Here's how the part is built. I have some questions about the finished solid (model axes, mm). Round coordinates to 2 decimals unless told otherwise and drop trailing zeros. Order: outer loops, then holes, each group sorted by start corner. A loop starts at its lowest first (then second) coordinate and runs counter-clockwise, first axis right, second up. Notation, with made-up numbers: M 51,27 L 109,27 A12 cw 109,32 Z; hole C 2,65 d5. An arc over 180 degrees is marked long. Write item = value, one per line. Start each with the question number.
Item 1: I'm going to push flat-ended pins straight in: P1, Ø3, axis at x = 7.5, z = 54.5, coming from the -Y side; P2, Ø2, axis at y = 10.5, z = 24.5, coming from the -X side; P3, Ø4, axis at x = 6, z = 10, coming from the +Y side. Where does each tip first touch, or does it pass through?
Item 2: Please list where these lines run through material, in increasing order: L1, parallel to Y at x = 0, z = 32; L2, parallel to Y at x = -8, z = 25; L3, parallel to X at y = -4, z = 72.
Item 3: We'd pull the mould along X, two halves only. Please class faces 1 (the face through (14, -14, 78.994)), 2 (the face through (-37.82, 1.66, 39.02)), 3 (the face through (-2.227, 16.964, 40.05)): pulls with the +X half, pulls with the -X half, needs draft (parallel to the pull), parting line crosses it, or undercut.
Item 4: I want a section at A-A, the plane x = 0. List the corners of the cut face in (y, z) for me, plus the area to 3 significant figures.
Item 5: I want a section at C-C, the plane z = 25. List the corners of the cut face in (x, y) for me, plus the area to 3 significant figures.
```python
from build123d import *

# Parameters (mm, degrees)
F0_R     = 37.855446
F1_DEPTH = 78.994
F2_R     = 5.08
F3_R     = 17.109797
F4_DEPTH = 118.11


with BuildPart() as f1:
    # F0 (on Top) → F1 (new body)
    with BuildSketch(Plane.XY):
        Circle(F0_R)
    extrude(amount=F1_DEPTH)

    # F2
    f2_edges = [f1.edges().sort_by_distance(p)[0] for p in [
        (37.855446, 0, 39.497),
        (-37.855446, 0, 0),
        (-37.855446, 0, 78.994),
    ]]
    fillet(f2_edges, radius=F2_R)

    # F3 (on face) → F4 (cut)
    with BuildSketch(Plane.XY.offset(78.994)):
        Circle(F3_R)
    extrude(amount=-F4_DEPTH, mode=Mode.SUBTRACT)


solid = f1.part
```
Filled in:
q1.P1 = -37.38
q1.P2 = -36.64
q1.P3 = 37.64
q2.L1 = -37.86 to -17.11, 17.11 to 37.86
q2.L2 = -37 to -15.12, 15.12 to 37
q2.L3 = -37.64 to -16.64, 16.64 to 37.64
q3.face_1 = needs draft
q3.face_2 = parting line crosses it
q3.face_3 = undercut
q4.outline = M -37.86,5.08 A5.08 ccw -32.78,0 L -17.11,0 L -17.11,78.99 L -32.78,78.99 A5.08 ccw -37.86,73.91 Z; M 17.11,0 L 32.78,0 A5.08 ccw 37.86,5.08 L 37.86,73.91 A5.08 ccw 32.78,78.99 L 17.11,78.99 Z
q4.area = 3,260 mm^2
q5.outline = C 0,0 d75.71; hole C 0,0 d34.22
q5.area = 3,580 mm^2
